```python
from build123d import *

# Parameters (mm, degrees)
SKETCH_1_R          = 1.585
EXTRUDE_1_DEPTH     = 2
SKETCH_2_R          = 5.2
EXTRUDE_2_DEPTH     = 7
SKETCH_3_R          = 1.585
CUT_EXTRUDE_1_DEPTH = 10


with BuildPart() as part:
    # 草图1 → 凸台-拉伸1 (new body)
    with BuildSketch(Plane(origin=(0, 0, 0), x_dir=(1, 0, 0), z_dir=(0, 1, 0))):
        Polygon((90, 10), (100, 0), (100, -10), (-90, -10), (-100, 0), (-100, 10), align=None)
        Circle(SKETCH_1_R, mode=Mode.SUBTRACT)
    extrude(amount=EXTRUDE_1_DEPTH)

    # 草图2 → 凸台-拉伸2 (add, symmetric)
    with BuildSketch(Plane.XZ):
        Circle(SKETCH_2_R)
    extrude(amount=EXTRUDE_2_DEPTH, both=True)

    # 草图3 → 切除-拉伸1 (cut)
    with BuildSketch(Plane(origin=(0, 7, 0), x_dir=(1, 0, 0), z_dir=(0, 1, 0))):
        Circle(SKETCH_3_R)
    extrude(amount=-CUT_EXTRUDE_1_DEPTH, mode=Mode.SUBTRACT)


solid = part.part
```
CAD build for the part. Positions are in the model's coordinates, mm. A direction names the side the tool comes from. Coordinates: 2 decimals unless noted, no trailing zeros. Write each loop counter-clockwise with the first axis right and the second up, starting at its lowest first coordinate (ties: lowest second). Pieces come first, ordered by that corner, then holes. Notation, with made-up numbers: (42, 8) -> (49, 8) arc R17 ccw to (49, 40) -> close; hole circle Ø9 at (-30.5, -1.5). An arc over 180 degrees is marked (long way). Return JSON: item names as keys, results as strings. Group by question number.
Q1. Cut at A-A, the plane y = 3.75. Give the cut face in (x, z) (3 decimals).
Q2. Flat gauge pins, fed straight in: pin 1 (2 mm diameter, centred on x = 12.5, z = 0.5, fed in from -Y); pin 2 (3 mm diameter, centred on x = 0, z = 0, fed in from +Y). Where does each tip first touch, or does it go through?
Q3. Cut at B-B, the plane x = -32. Give the cut face in (y, z), then the cut area to 3 significant figures.
Q4. Drill centre lines: line 1 (X direction, y = 1.75, z = 0) (3 decimals); line 2 (Z direction, x = 0, y = 5.25) (3 decimals); line 3 (X direction, y = -1, z = 0.25). Where is each one in solid material? Low to high.
Q5. Which spindle directions (+Z, -Z, +X, -X, +Y, -Y) get a long thin tool onto all of the face, cutting with end or side? Do faces 5 (the face through (-0.677, -3.549, 5.156)), 6 (the face through (0, -7, 0)). Say none if no direction does.
Q6. Pull direction Z, two halves, no side cores. Call faces 1 (the face through (-0.677, 4.465, 5.156)), 2 (the face through (-1.23, 7, 1.23)), 3 (the face through (-1.26, 2.07, 0.96)), 4 (the face through (0, -3, 0)): released by +Z, released by -Z, zero draft, split by the parting line, or undercut.
Returned:
{
 "1": {"outline": "circle Ø10.4 at (0, 0); hole circle Ø3.17 at (0, 0)"},
 "2": {"pin 1": "stops at y = 0", "pin 2": "stops at y = -3"},
 "3": {"outline": "(0, -10) -> (2, -10) -> (2, 10) -> (0, 10) -> close", "area": "40.0 mm2"},
 "4": {"line 1": "x = -100 to -1.585, 1.585 to 100", "line 2": "z = -5.2 to -1.585, 1.585 to 5.2", "line 3": "x = -5.19 to -1.57, 1.57 to 5.19"},
 "5": {"face 5": "-Y", "face 6": "+Z, -Z, +X, -X, -Y"},
 "6": {"face 1": "split by the parting line", "face 2": "zero draft", "face 3": "undercut", "face 4": "undercut"}
}
